Geometry check sheet. Reference: the model listing, model coordinates, mm. Face numbers are marked on the shaded views. A direction names the side the tool comes from. Coordinates: 2 decimals unless noted, no trailing zeros. Write each loop counter-clockwise with the first axis right and the second up, starting at its lowest first coordinate (ties: lowest second). Pieces come first, ordered by that corner, then holes. Notation, with made-up numbers: (-33.75, -9) -> (-22.75, -9) arc R35 cw to (-22.75, 28) -> close; hole circle Ø8 at (-16.5, 65.25). An arc over 180 degrees is marked (long way). Answer in a Markdown table with one row per item. Add a question column.
1. Set-up check for the marked faces 5 and 6: record each of +Z, -Z, +X, -X, +Y, -Y from which the full face is reachable in a straight line by a thin tool's end or side.
2. Cross-section at B-B on x = 1.05. Record the cut outline in (y, z).
3. Mould release check, pull along Z, two halves, no side actions. Record for the marked faces 1, 2, 3 and 4: pulls with the +Z half, pulls with the -Z half, needs draft (parallel to the pull), parting line crosses it, or undercut.
4. Cross-section at D-D on x = 3.6. Record the cut outline in (y, z), and give its area (3 significant figures).
5. Cross-section at A-A on y = -1.5. Record the cut outline in (x, z), and give its area (3 significant figures).
6. Depth check by flat-ended pin: P1, Ø2.5, axis at y = -3, z = -14, coming from the +X side; P2, Ø1, axis at x = 0.5, z = -10, coming from the +Y side; P3, Ø2.5, axis at y = -1.5, z = -25, coming from the -X side. Enter the tip coordinate at first touch or a pass-through.
7. Cross-section at C-C on z = -15.5. Record the cut outline in (x, y).
8. Scan lines: L1, parallel to Y at x = 0.8, z = 0; L2, parallel to X at y = -5, z = -16; L3, parallel to Z at x = 0.6, y = -2. Record each from-to range of solid material in increasing order. Write a range as from..to.
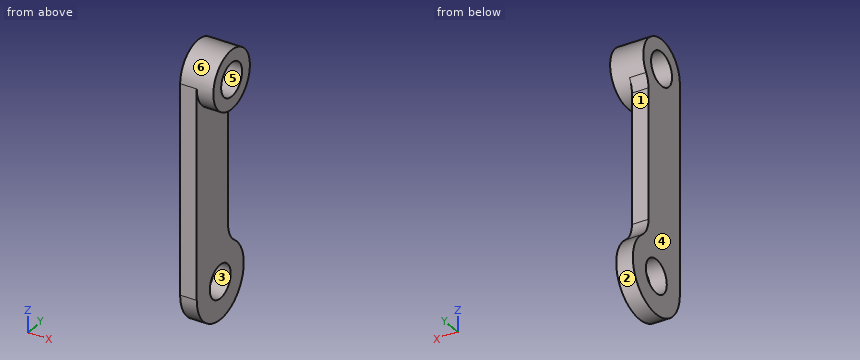
```python
from build123d import *

# Parameters (mm, degrees)
SKETCH_1_R               = 3.5
SKETCH_1_R_2             = 4.5
SKETCH_1_W               = 25
SKETCH_1_H               = 6
EXTRUDE_1_DEPTH          = 2
EXTRUDE_START            = 2
SKETCH_1_5_R             = 3.5
EXTRUDE_3_DEPTH          = 2
CUT_EXTRUDE_2_DEPTH      = 31.368569278
CUT_EXTRUDE_2_DEPTH_BACK = 31.368569278
SKETCH_1_4_R             = 2
FILLET_1_R               = 3


with BuildPart() as part:
    # 草图1 → 凸台-拉伸1 (new body)
    with BuildSketch(Plane(origin=(0, 0, 0), x_dir=(0, 0, -1), z_dir=(1, 0, 0))):
        with Locations((0, -2.5)):
            Circle(SKETCH_1_R)
        with Locations((25, -1.5)):
            Circle(SKETCH_1_R_2)
        with Locations((12.5, -3)):
            Rectangle(SKETCH_1_W, SKETCH_1_H)
    extrude(amount=EXTRUDE_1_DEPTH)

    # 草图1<5> → 凸台-拉伸3 (add)
    with BuildSketch(Plane(origin=(0, 0, 0), x_dir=(0, 0, -1), z_dir=(1, 0, 0)).offset(EXTRUDE_START)):
        with Locations(Location((0, -2.5, 0), (0, 0, 270))):
            Circle(SKETCH_1_5_R)
    extrude(amount=EXTRUDE_3_DEPTH)

    # 草图1<4> → 切除-拉伸2 (cut, two sides: drawn at the far end of the back side and taken through both)
    with BuildSketch(Plane(origin=(0, 0, 0), x_dir=(0, 0, -1), z_dir=(1, 0, 0)).offset(-CUT_EXTRUDE_2_DEPTH_BACK)):
        with Locations((0, -2.5)):
            Circle(SKETCH_1_4_R)
        with Locations((25, -1.5)):
            Circle(SKETCH_1_4_R)
    extrude(amount=CUT_EXTRUDE_2_DEPTH + CUT_EXTRUDE_2_DEPTH_BACK, mode=Mode.SUBTRACT)

    # 圆角1
    fillet_1_edges = [part.edges().sort_by_distance(p)[0] for p in [
        (1, 0, -20.757359313),
        (1, 0, -2.449489743),
    ]]
    fillet(fillet_1_edges, radius=FILLET_1_R)


solid = part.part
```
Results found:
| question | item | result |
|---|---|---|
| 1 | face 5 | +X, -X |
| 1 | face 6 | +X |
| 2 | outline | (-6, -25) arc R4.5 ccw (long way) to (1.2, -21.4) arc R3 cw to (0, -19) -> (0, -3.46) arc R3 cw to (0.46, -1.87) arc R3.5 ccw (long way) to (-6, 0) -> close; hole circle Ø4 at (-2.5, 0); hole circle Ø4 at (-1.5, -25) |
| 3 | face 1 | undercut |
| 3 | face 2 | parting line crosses it |
| 3 | face 3 | undercut |
| 3 | face 4 | needs draft |
| 4 | outline | circle Ø7 at (-2.5, 0); hole circle Ø4 at (-2.5, 0) |
| 4 | area | 25.9 mm^2 |
| 5 | outline | (0, -29.5) -> (2, -29.5) -> (2, -27) -> (0, -27) -> close; (0, -23) -> (2, -23) -> (2, -3.35) -> (4, -3.35) -> (4, -1.73) -> (0, -1.73) -> close; (0, 1.73) -> (4, 1.73) -> (4, 3.35) -> (0, 3.35) -> close |
| 5 | area | 57.3 mm^2 |
| 6 | P1 | stops at x = 2 |
| 6 | P2 | stops at y = 0 |
| 6 | P3 | passes through |
| 7 | outline | (0, -6) -> (2, -6) -> (2, 0) -> (0, 0) -> close |
| 8 | L1 | y = -6..-4.5, -0.5..1 |
| 8 | L2 | x = 0..2 |
| 8 | L3 | z = -29.47..-26.94, -23.06..-1.94, 1.94..3.46 |
